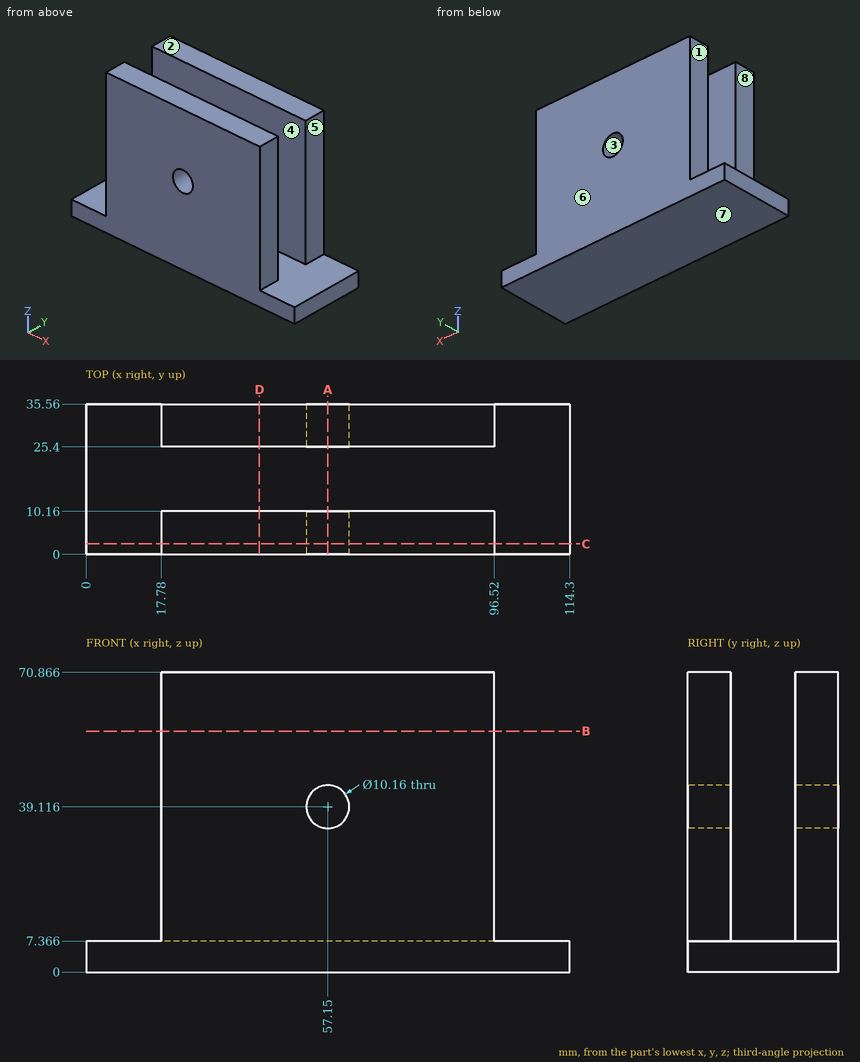
Here's the drawing with two shaded views (mm, measured from the low corner). I have some questions. A direction names the side the tool comes from. Round coordinates to 2 decimals unless told otherwise and drop trailing zeros. Write each loop counter-clockwise with the first axis right and the second up, starting at its lowest first coordinate (ties: lowest second). Pieces come first, ordered by that corner, then holes.
(1) Which directions (+Z, -Z, +X, -X, +Y, -Y) give clear straight access to the entire face, cutting with the end or side of a thin tool? Please do the marked faces 4, 5, 6, 7 and 8.
Findings below:
face 4: +Z, +X, -X
face 5: +Z, +X, +Y, -Y
face 6: +Z, -Z, +X, -X, +Y
face 7: -Z, +X, -X, +Y, -Y
face 8: +Z, -X, +Y, -Y
(2) Suppose I cut it at B-B on z = 57. Write out the boundary of the cut face in (x, y), and give its area (3 significant figures).
Findings below:
outline: (17.78, 0) - (96.52, 0) - (96.52, 10.16) - (17.78, 10.16) - close; (17.78, 25.4) - (96.52, 25.4) - (96.52, 35.56) - (17.78, 35.56) - close
area: 1,600 mm2
(3) Thinking about a two-plate mould opening in Z: for the marked faces 1, 2 and 3, which applies, +Z half, -Z half, draft (parallel to the pull), parting line (faces both ways), or undercut?
Findings below:
face 1: draft
face 2: +Z half
face 3: undercut
(4) Suppose I cut it at D-D on x = 41. Write out the boundary of the cut face in (y, z), and give its area (3 significant figures).
Findings below:
outline: (0, 0) - (35.56, 0) - (35.56, 70.87) - (25.4, 70.87) - (25.4, 7.37) - (10.16, 7.37) - (10.16, 70.87) - (0, 70.87) - close
area: 1,550 mm2
(5) If I drill on probe 1 along Y at (x, z) = (71, 54); probe 2 along Z at (x, y) = (57, 6); probe 3 along X at (y, z) = (5, 25.5), over which ranges is the centre line in solid material (lowest first)?
Findings below:
probe 1: y = 0 to 10.16, 25.4 to 35.56
probe 2: z = 0 to 34.04, 44.19 to 70.87
probe 3: x = 17.78 to 96.52
(6) Suppose I cut it at C-C on y = 2.5. Write out the boundary of the cut face in (x, z).
Findings below:
outline: (0, 0) - (114.3, 0) - (114.3, 7.37) - (96.52, 7.37) - (96.52, 70.87) - (17.78, 70.87) - (17.78, 7.37) - (0, 7.37) - close; hole circle Ø10.16 at (57.15, 39.12)
(7) For pin 1 (11.5 mm diameter, centred on x = 57.15, z = 39.116, fed in from +Y); pin 2 (12 mm diameter, centred on y = 29, z = 24, fed in from +X); pin 3 (3 mm diameter, centred on y = 5.5, z = 52.5, fed in from -X); pin 4 (1 mm diameter, centred on x = 92.5, y = 22, fed in from +Z), each with a flat end and sliding along its axis, tell me the tip position at first contact or that it passes through.
Findings below:
pin 1: stops at y = 35.56
pin 2: stops at x = 96.52
pin 3: stops at x = 17.78
pin 4: stops at z = 7.37
(8) Suppose I cut it at A-A on x = 57.15. Write out the boundary of the cut face in (y, z), and give its area (3 significant figures).
Findings below:
outline: (0, 0) - (35.56, 0) - (35.56, 34.04) - (25.4, 34.04) - (25.4, 7.37) - (10.16, 7.37) - (10.16, 34.04) - (0, 34.04) - close; (0, 44.2) - (10.16, 44.2) - (10.16, 70.87) - (0, 70.87) - close; (25.4, 44.2) - (35.56, 44.2) - (35.56, 70.87) - (25.4, 70.87) - close
area: 1,350 mm2
